Design review of the part built by this model. Coordinates are the model's own, in mm. Face numbers are marked on the shaded views. A direction names the side the tool comes from. Give positions to 0.01 mm unless a question says otherwise; leave off trailing zeros. Loops run counter-clockwise (first coordinate to the right, second up) from the corner with the lowest first, then second, coordinate; pieces in that order, holes last. Notation, with made-up numbers: M 13,55 L 44,55 A10 ccw 44,61 Z; hole C 62,84.25 d1. An arc over 180 degrees is marked long. Use CSV: the item, a comma, the result in double quotes.
from build123d import *

# Parameters (mm, degrees)
BOSS_EXTRUDE1_DEPTH = 6.604
CUT_EXTRUDE1_DEPTH  = 7.604
SKETCH3_W           = 6.35
SKETCH3_H           = 4.826
BOSS_EXTRUDE2_DEPTH = 6.604
FILLET1_R           = 12.7


with BuildPart() as part:
    # Sketch1 → Boss-Extrude1 (new body)
    with BuildSketch(Plane.XY):
        Polygon((-6.858, 0), (-6.858, -9.525), (11.557, -9.525), (11.557, -1.905), (17.907, -1.905), (17.907, -27.305), (-66.802, -27.305), (-66.802, -1.905), (-12.7, -1.905), (-12.7, 0), align=None)
    extrude(amount=BOSS_EXTRUDE1_DEPTH)

    # Sketch2 → Cut-Extrude1 (cut, through all)
    with BuildSketch(Plane.XY.offset(6.604)):
        Polygon((-53.0098, -1.905), (-53.0098, -8.255), (-55.2958, -8.255), (-55.2958, -14.1986), (-53.0098, -14.1986), (-53.0098, -17.399), (-48.8442, -17.399), (-48.8442, -14.1986), (-46.5582, -14.1986), (-46.5582, -8.255), (-48.8442, -8.255), (-48.8442, -1.905), align=None)
        Polygon((-33.9598, -1.905), (-33.9598, -8.255), (-36.2458, -8.255), (-36.2458, -14.1986), (-33.9598, -14.1986), (-33.9598, -17.399), (-29.7942, -17.399), (-29.7942, -14.1986), (-27.5082, -14.1986), (-27.5082, -8.255), (-29.7942, -8.255), (-29.7942, -1.905), align=None)
    extrude(amount=-CUT_EXTRUDE1_DEPTH, mode=Mode.SUBTRACT)

    # Sketch3 → Boss-Extrude2 (add)
    with BuildSketch(Plane.XY.offset(6.604)):
        with Locations((-60.452, 0.508)):
            Rectangle(SKETCH3_W, SKETCH3_H)
        with Locations((-41.402, 0.508)):
            Rectangle(SKETCH3_W, SKETCH3_H)
        with Locations((-22.352, 0.508)):
            Rectangle(SKETCH3_W, SKETCH3_H)
    extrude(amount=-BOSS_EXTRUDE2_DEPTH)

    # Fillet1
    fillet1_edges = [part.edges().sort_by_distance(p)[0] for p in [
        (17.907, -27.305, 3.302),
        (-66.802, -27.305, 3.302),
    ]]
    fillet(fillet1_edges, radius=FILLET1_R)


solid = part.part
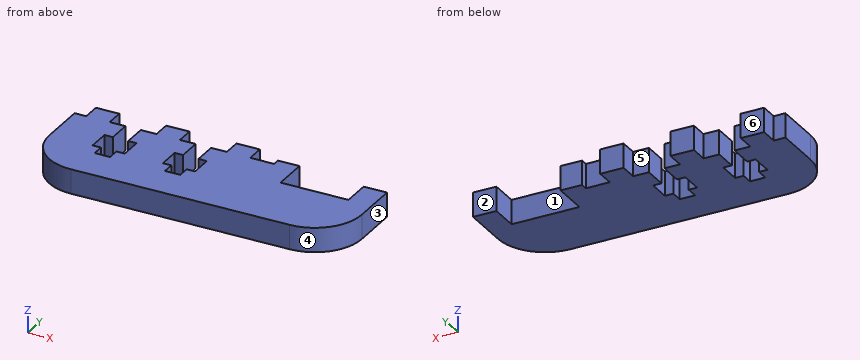
(1) We need section B-B on y = 1.5. State the section outline as (x, z) points, then the cut area to 3 significant figures.
A:
outline,"M -63.63,0 L -57.28,0 L -57.28,6.6 L -63.63,6.6 Z; M -44.58,0 L -38.23,0 L -38.23,6.6 L -44.58,6.6 Z; M -25.53,0 L -19.18,0 L -19.18,6.6 L -25.53,6.6 Z"
area,"126 mm²"
(2) The part is to be moulded in two halves that separate along X. For the marked faces 4, 5 and 6, say which applies: released by +X, released by -X, zero draft, split by the parting line, or undercut.
A:
face 4,"released by +X"
face 5,"undercut"
face 6,"zero draft"
(3) Wall thickness on line 1 along X through (y, z) = (-14.5, 3.25); line 2 along X through (y, z) = (-2.5, 4.25); line 3 along X through (y, z) = (-12, 2.25): over which ranges is each line inside the solid? List them lowest first. Write a range as [from, to].
A:
line 1,"[-66.8, -53.01], [-48.84, -33.96], [-29.79, 17.91]"
line 2,"[-66.8, -53.01], [-48.84, -33.96], [-29.79, -6.86], [11.56, 17.91]"
line 3,"[-66.8, -55.3], [-46.56, -36.25], [-27.51, 17.91]"
(4) Machinability: for the marked faces 1, 2 and 3, which of the approach directions +Z, -Z, +X, -X, +Y, -Y give a long, thin tool a straight path to every point of the face, cutting with its end or side? Answer none if there is none.
A:
face 1,"+Z, -Z, +Y"
face 2,"+Z, -Z, +X, +Y"
face 3,"+Z, -Z, +X, +Y, -Y"
(5) We need section C-C on x = -8.5. State the section outline as (y, z) points (3 decimals).
A:
outline,"M -27.305,0 L 0,0 L 0,6.604 L -27.305,6.604 Z"
(6) We need section A-A on y = -5. State the section outline as (x, z) points, then the cut area to 3 significant figures.
A:
outline,"M -66.8,0 L -53.01,0 L -53.01,6.6 L -66.8,6.6 Z; M -48.84,0 L -33.96,0 L -33.96,6.6 L -48.84,6.6 Z; M -29.79,0 L -6.86,0 L -6.86,6.6 L -29.79,6.6 Z; M 11.56,0 L 17.91,0 L 17.91,6.6 L 11.56,6.6 Z"
area,"383 mm²"
(7) We need section D-D on x = -31. State the section outline as (y, z) points (3 decimals).
A:
outline,"M -27.305,0 L -17.399,0 L -17.399,6.604 L -27.305,6.604 Z"
(8) Clearance check with flat-ended pins moving along their axes: P1, Ø2, axis at x = -46.5, z = 4, coming from the +Y side (3 decimals); P2, Ø1, axis at y = -16.5, z = 3, coming from the +X side; P3, Ø1.2, axis at x = -32.5, z = 3.5, coming from the +Y side. State where each tip first meets the part, or that it passes through.
A:
P1,"y = -1.905"
P2,"x = 17.83"
P3,"y = -17.4"
